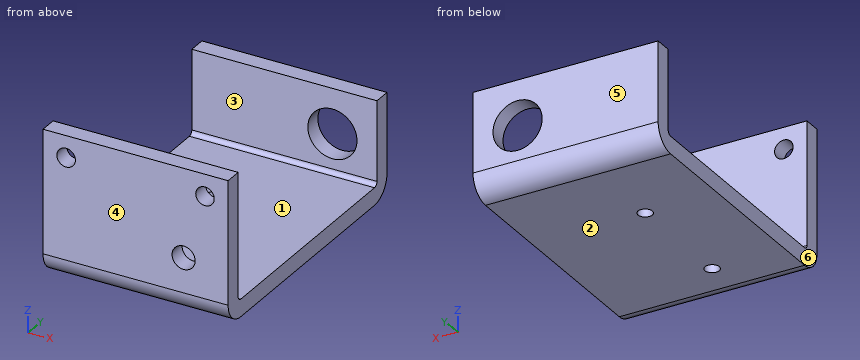
```python
from build123d import *

# Parameters (mm, degrees)
SKETCH1_W                        = 32
SKETCH1_H                        = 25
BASE_FLANGE1_DEPTH               = 3
EDGE_FLANGE1_STRIP_W             = 13.4732
EDGE_FLANGE1_STRIP_H             = 3
EDGE_FLANGE1_STRIP_CUT_DEPTH     = 32
EDGE_FLANGE1_DEPTH               = 32
EDGE_FLANGE2_STRIP_W             = 13.4732
EDGE_FLANGE2_STRIP_H             = 3
EDGE_FLANGE2_STRIP_CUT_DEPTH     = 32
EDGE_FLANGE2_DEPTH               = 32
TAP_DRILL_FOR_M3X0_5_TAP1_D      = 2.5
TAP_DRILL_FOR_M10X1_5_TAP2_D     = 8.5
TAP_DRILL_FOR_M10X1_5_TAP2_DEPTH = 3
M3_CLEARANCE_HOLE1_D             = 3.2
F_4_0_4_DIAMETER_HOLE1_D         = 4


# Sheet-metal steps are written as plain solids
with BuildPart() as part:
    # Sketch1 → Base-Flange1 (new body)
    with BuildSketch(Plane(origin=(0, 0, 0), x_dir=(1, 0, 0), z_dir=(0, 1, 0))):
        Rectangle(SKETCH1_W, SKETCH1_H)
    extrude(amount=-BASE_FLANGE1_DEPTH)

    # Edge-Flange1 strip (across the edge) → Edge-Flange1 strip cut (cut)
    with BuildSketch(Plane(origin=(16, 0, -12.5), x_dir=(0, 0, 1), z_dir=(-1, 0, 0))):
        with Locations((-3, -1.5)):
            Rectangle(EDGE_FLANGE1_STRIP_W, EDGE_FLANGE1_STRIP_H)
    extrude(amount=EDGE_FLANGE1_STRIP_CUT_DEPTH, mode=Mode.SUBTRACT)

    # Edge-Flange1 section (across the edge) → Edge-Flange1 (add)
    with BuildSketch(Plane(origin=(16, 0, -12.5), x_dir=(0, 0, 1), z_dir=(-1, 0, 0))):
        with BuildLine():
            Line((0, 0.7366), (0, 44.5))
            Line((0, 44.5), (3, 44.5))
            Line((3, 44.5), (3, 0.7366))
            ThreePointArc((3, 0.7366), (3.215745145, 0.215745145), (3.7366, 0))
            Line((3.7366, 0), (3.7366, -3))
            ThreePointArc((3.7366, -3), (1.094424801, -1.905575199), (0, 0.7366))
        make_face()
    extrude(amount=EDGE_FLANGE1_DEPTH)

    # Edge-Flange2 strip (across the edge) → Edge-Flange2 strip cut (cut)
    with BuildSketch(Plane(origin=(16, 44.5, -9.5), x_dir=(0, -1, 0), z_dir=(-1, 0, 0))):
        with Locations((-3, -1.5)):
            Rectangle(EDGE_FLANGE2_STRIP_W, EDGE_FLANGE2_STRIP_H)
    extrude(amount=EDGE_FLANGE2_STRIP_CUT_DEPTH, mode=Mode.SUBTRACT)

    # Edge-Flange2 section (across the edge) → Edge-Flange2 (add)
    with BuildSketch(Plane(origin=(16, 44.5, -9.5), x_dir=(0, -1, 0), z_dir=(-1, 0, 0))):
        with BuildLine():
            Line((0, 0.7366), (0, 14.5))
            Line((0, 14.5), (3, 14.5))
            Line((3, 14.5), (3, 0.7366))
            ThreePointArc((3, 0.7366), (3.215745145, 0.215745145), (3.7366, 0))
            Line((3.7366, 0), (3.7366, -3))
            ThreePointArc((3.7366, -3), (1.094424801, -1.905575199), (0, 0.7366))
        make_face()
    extrude(amount=EDGE_FLANGE2_DEPTH)

    # Tap Drill for M3x0.5 Tap1 (through all)
    with Locations(Plane.XY.offset(-9.5)):
        with Locations((-3.5, 6.7366), (-3.5, 26.7366)):
            Hole(TAP_DRILL_FOR_M3X0_5_TAP1_D / 2)

    # Tap Drill for M10x1.5 Tap2
    with Locations(Plane(origin=(0, 44.5, 0), x_dir=(1, 0, 0), z_dir=(0, 1, 0))):
        with Locations((8.3, 2.7634)):
            Hole(TAP_DRILL_FOR_M10X1_5_TAP2_D / 2, depth=TAP_DRILL_FOR_M10X1_5_TAP2_DEPTH)

    # M3 Clearance Hole1 (through all)
    with Locations(Plane(origin=(0, 0, 0), x_dir=(1, 0, 0), z_dir=(0, 1, 0))):
        with Locations((-12, -8.7366), (12, -8.7366)):
            Hole(M3_CLEARANCE_HOLE1_D / 2)

    # Ø4.0 (4) Diameter Hole1 (through all)
    with Locations(Plane(origin=(0, 0, 0), x_dir=(1, 0, 0), z_dir=(0, 1, 0))):
        with Locations((8.3, 2.7634)):
            Hole(F_4_0_4_DIAMETER_HOLE1_D / 2)


solid = part.part
```
Here's how the part is built. I have some questions about the finished solid (model axes, mm). Face numbers are marked on the shaded views. A direction names the side the tool comes from. Coordinates: 2 decimals unless noted, no trailing zeros. Order: outer loops, then holes, each group sorted by start corner. A loop starts at its lowest first (then second) coordinate and runs counter-clockwise, first axis right, second up.
Item 1: If we section it at D-D, the plane z = 8: List the corners of the cut face in (x, y) for me, then the cut area to 3 significant figures.
Response values:
outline: (-16, -3) - (-13.42, -3) - (-13.42, 0) - (-16, 0) - close; (-10.58, -3) - (10.58, -3) - (10.58, 0) - (-10.58, 0) - close; (13.42, -3) - (16, -3) - (16, 0) - (13.42, 0) - close
area: 79.0 mm2
Item 2: Which directions (+Z, -Z, +X, -X, +Y, -Y) give clear straight access to the entire face, cutting with the end or side of a thin tool? Please do the marked faces 1 and 2.
Response values:
face 1: +Z, +X, -X
face 2: -Z, +X, -X, +Y, -Y
Item 3: I'm going to push flat-ended pins straight in: pin 1 Ø1.9 at (x, z) = (-12, 8.74) entering from -Y; pin 2 Ø3 at (x, y) = (-3.5, 6.74) entering from +Z; pin 3 Ø3 at (x, z) = (-8.5, 8.5) entering from +Y; pin 4 Ø2.5 at (x, y) = (-6, 42.5) entering from +Z. Where does each tip first touch, or does it pass through?
Response values:
pin 1: passes through
pin 2: stops at z = -9.5
pin 3: stops at y = 0
pin 4: stops at z = 5
Item 4: If we section it at B-B, the plane z = 4.25: List the corners of the cut face in (x, y) for me, then the cut area to 3 significant figures.
Response values:
outline: (-16, -3) - (16, -3) - (16, 0) - (-16, 0) - close; (-16, 41.5) - (16, 41.5) - (16, 44.5) - (-16, 44.5) - close
area: 192 mm2
Item 5: Thinking about a two-plate mould opening in Y: for the marked faces 3, 4, 5 and 6, which applies, pulls with the +Y half, pulls with the -Y half, needs draft (parallel to the pull), parting line crosses it, or undercut?
Response values:
face 3: undercut
face 4: pulls with the -Y half
face 5: pulls with the +Y half
face 6: needs draft
Item 6: If we section it at C-C, the plane x = -12: List the corners of the cut face in (y, z) for me.
Response values:
outline: (-3, -8.76) arc R3.74 ccw to (0.74, -12.5) - (40.76, -12.5) arc R3.74 ccw to (44.5, -8.76) - (44.5, 5) - (41.5, 5) - (41.5, -8.76) arc R0.74 cw to (40.76, -9.5) - (0.74, -9.5) arc R0.74 cw to (0, -8.76) - (0, 7.14) - (-3, 7.14) - close; (-3, 10.34) - (0, 10.34) - (0, 12.5) - (-3, 12.5) - close
Item 7: I need wall thicknesses on probe 1 along Y at (x, z) = (-4, -3.5); probe 2 along Y at (x, z) = (-3.5, -10.1); probe 3 along Z at (x, y) = (0.5, 6.5). Which ranges of each line are inside material? Lowest first, please.
Response values:
probe 1: y = -3 to 0, 41.5 to 44.5
probe 2: y = -2.75 to 5.49, 7.99 to 25.49, 27.99 to 44.25
probe 3: z = -12.5 to -9.5
Item 8: If we section it at A-A, the plane x = 8.3: List the corners of the cut face in (y, z) for me.
Response values:
outline: (-3, -8.76) arc R3.74 ccw to (0.74, -12.5) - (40.76, -12.5) arc R3.74 ccw to (44.5, -8.76) - (44.5, -7.01) - (41.5, -7.01) - (41.5, -8.76) arc R0.74 cw to (40.76, -9.5) - (0.74, -9.5) arc R0.74 cw to (0, -8.76) - (0, -4.76) - (-3, -4.76) - close; (-3, -0.76) - (0, -0.76) - (0, 12.5) - (-3, 12.5) - close; (41.5, 1.49) - (44.5, 1.49) - (44.5, 5) - (41.5, 5) - close
